The model under review builds one solid part; all positions refer to its coordinate system, in mm. Coordinates: 2 decimals unless noted, no trailing zeros. Answer in a Markdown table with one row per item.
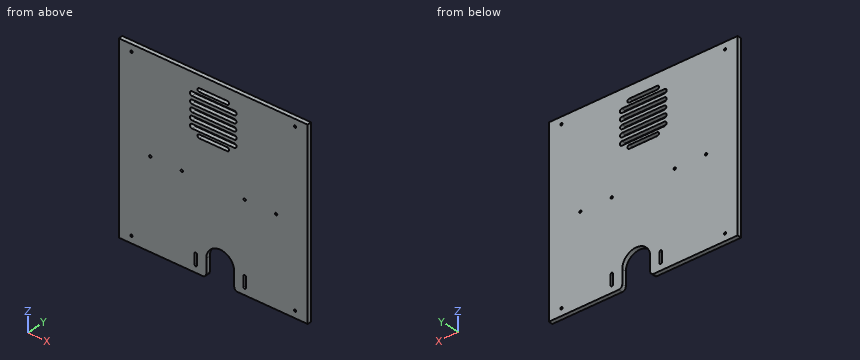
```python
from build123d import *

# Parameters (mm, degrees)
SKETCH1_R               = 1.6
BOSS_EXTRUDE1_DEPTH     = 6
CUT_EXTRUDE1_DEPTH      = 203.20197823
CUT_EXTRUDE1_DEPTH_BACK = 203.20197823
SKETCH4_R               = 1.6
CUT_EXTRUDE2_DEPTH      = 10
CUT_EXTRUDE3_DEPTH      = 10
FILLET1_R               = 5
CUT_EXTRUDE4_DEPTH      = 10
CUT_EXTRUDE4_DEPTH_BACK = 10


with BuildPart() as part:
    # Sketch1 → Boss-Extrude1 (new body)
    with BuildSketch(Plane(origin=(0, 0, 0), x_dir=(1, 0, 0), z_dir=(0, 1, 0))):
        Polygon((-145, 120), (125, 120), (125, -100.8), (125, -140.8), (-145, -140.8), (-145, -100.8), align=None)
        with Locations(Location((-100, -5, 0), (0, 0, 270))):
            Circle(SKETCH1_R, mode=Mode.SUBTRACT)
        with Locations(Location((80, -5, 0), (0, 0, 270))):
            Circle(SKETCH1_R, mode=Mode.SUBTRACT)
        with Locations(Location((-55, -5, 0), (0, 0, 270))):
            Circle(SKETCH1_R, mode=Mode.SUBTRACT)
        with Locations(Location((35, -5, 0), (0, 0, 270))):
            Circle(SKETCH1_R, mode=Mode.SUBTRACT)
    extrude(amount=BOSS_EXTRUDE1_DEPTH)

    # Sketch3 → Cut-Extrude1 (cut, two sides: drawn at the far end of the back side and taken through both)
    with BuildSketch(Plane(origin=(0, 6, 0), x_dir=(1, 0, 0), z_dir=(0, 1, 0)).offset(-CUT_EXTRUDE1_DEPTH_BACK)):
        with BuildLine():
            Line((-20, 95), (-20, 120))
            Line((-20, 120), (20, 120))
            Line((20, 120), (20, 95))
            ThreePointArc((20, 95), (0, 75), (-20, 95))
        make_face()
    extrude(amount=CUT_EXTRUDE1_DEPTH + CUT_EXTRUDE1_DEPTH_BACK, mode=Mode.SUBTRACT)

    # Sketch4 → Cut-Extrude2 (cut)
    with BuildSketch(Plane.XZ):
        with Locations(Location((107, -110, 0), (0, 0, 270))):
            Circle(SKETCH4_R)
        with Locations(Location((-127, -110, 0), (0, 0, 270))):
            Circle(SKETCH4_R)
        with Locations(Location((107, 130.8, 0), (0, 0, 270))):
            Circle(SKETCH4_R)
        with Locations(Location((-127, 130.8, 0), (0, 0, 270))):
            Circle(SKETCH4_R)
    extrude(amount=-CUT_EXTRUDE2_DEPTH, mode=Mode.SUBTRACT)

    # Sketch5 → Cut-Extrude3 (cut)
    with BuildSketch(Plane(origin=(0, 6, 0), x_dir=(1, 0, 0), z_dir=(0, 1, 0))):
        with BuildLine():
            Line((-33.4, 110), (-33.4, 95))
            ThreePointArc((-33.4, 95), (-35, 93.4), (-36.6, 95))
            Line((-36.6, 95), (-36.6, 110))
            ThreePointArc((-36.6, 110), (-35, 111.6), (-33.4, 110))
        make_face()
        with BuildLine():
            Line((33.4, 110), (33.4, 95))
            ThreePointArc((33.4, 95), (35, 93.4), (36.6, 95))
            Line((36.6, 95), (36.6, 110))
            ThreePointArc((36.6, 110), (35, 111.6), (33.4, 110))
        make_face()
    extrude(amount=-CUT_EXTRUDE3_DEPTH, mode=Mode.SUBTRACT)

    # Fillet1
    fillet1_edges = [part.edges().sort_by_distance(p)[0] for p in [
        (-20, 3, -120),
        (20, 3, -120),
    ]]
    fillet(fillet1_edges, radius=FILLET1_R)

    # Sketch6 → Cut-Extrude4 (cut, two sides: drawn at the far end of the back side and taken through both)
    with BuildSketch(Plane.XZ.offset(-CUT_EXTRUDE4_DEPTH_BACK)):
        with BuildLine():
            Line((10, 58.021465569), (-30, 58.021465569))
            ThreePointArc((-30, 58.021465569), (-32.570860459, 60.592326028), (-30, 63.163186487))
            Line((-30, 63.163186487), (10, 63.163186487))
            ThreePointArc((10, 63.163186487), (12.570860459, 60.592326028), (10, 58.021465569))
        make_face()
        with BuildLine():
            Line((20.436008981, 66.571059525), (-40.436008981, 66.571059525))
            ThreePointArc((-40.436008981, 66.571059525), (-43.436008981, 69.571059525), (-40.436008981, 72.571059525))
            Line((-40.436008981, 72.571059525), (20.436008981, 72.571059525))
            ThreePointArc((20.436008981, 72.571059525), (23.436008981, 69.571059525), (20.436008981, 66.571059525))
        make_face()
        with BuildLine():
            Line((20.316760433, 77.325947728), (-40.316760433, 77.325947728))
            ThreePointArc((-40.316760433, 77.325947728), (-43.316760433, 80.325947728), (-40.316760433, 83.325947728))
            Line((-40.316760433, 83.325947728), (20.316760433, 83.325947728))
            ThreePointArc((20.316760433, 83.325947728), (23.316760433, 80.325947728), (20.316760433, 77.325947728))
        make_face()
        with BuildLine():
            Line((-30, 123.777281933), (10, 123.777281933))
            ThreePointArc((10, 123.777281933), (12.570860459, 121.206421475), (10, 118.635561016))
            Line((10, 118.635561016), (-30, 118.635561016))
            ThreePointArc((-30, 118.635561016), (-32.570860459, 121.206421475), (-30, 123.777281933))
        make_face()
        with BuildLine():
            Line((-40.436008981, 115.227687978), (20.436008981, 115.227687978))
            ThreePointArc((20.436008981, 115.227687978), (23.436008981, 112.227687978), (20.436008981, 109.227687978))
            Line((20.436008981, 109.227687978), (-40.436008981, 109.227687978))
            ThreePointArc((-40.436008981, 109.227687978), (-43.436008981, 112.227687978), (-40.436008981, 115.227687978))
        make_face()
        with BuildLine():
            Line((-40.316760433, 104.472799775), (20.316760433, 104.472799775))
            ThreePointArc((20.316760433, 104.472799775), (23.316760433, 101.472799775), (20.316760433, 98.472799775))
            Line((20.316760433, 98.472799775), (-40.316760433, 98.472799775))
            ThreePointArc((-40.316760433, 98.472799775), (-43.316760433, 101.472799775), (-40.316760433, 104.472799775))
        make_face()
        with BuildLine():
            Line((20, 87.899373751), (-40, 87.899373751))
            ThreePointArc((-40, 87.899373751), (-43, 90.899373751), (-40, 93.899373751))
            Line((-40, 93.899373751), (20, 93.899373751))
            ThreePointArc((20, 93.899373751), (23, 90.899373751), (20, 87.899373751))
        make_face()
    extrude(amount=CUT_EXTRUDE4_DEPTH + CUT_EXTRUDE4_DEPTH_BACK, mode=Mode.SUBTRACT)


solid = part.part
```
Item 1: Clearance check with a flat-ended pin moving along its axis: pin 1 Ø3 at (x, z) = (-127, -110) entering from -Y. State where the tip first meets the part, or that it passes through.
Check values:
| item | result |
|---|---|
| pin 1 | through |
Item 2: We need section A-A, the plane x = -7. State how many separate pieces and enclosed holes the cut face has, then the cut area to 3 significant figures.
Check values:
| item | result |
|---|---|
| separate pieces | 8 |
| enclosed holes | 0 |
| area | 1,060 mm^2 |
Item 3: To check wall thickness, follow line 1 (X direction, y = 1.2, z = -110); line 2 (X direction, y = 4.1, z = 130.8); line 3 (Z direction, x = 107, y = 4.7). State the ranges of each line that lie inside material, in increasing order. Write a range as from..to.
Check values:
| item | result |
|---|---|
| line 1 | -145..-128.6, -125.4..-36.6, -33.4..-20, 20..33.4, 36.6..105.4, 108.6..125 |
| line 2 | -145..-128.6, -125.4..105.4, 108.6..125 |
| line 3 | -120..-111.6, -108.4..129.2, 132.4..140.8 |
